Can you work these out from the model? Positions are in its coordinate system, mm. Face numbers are marked on the shaded views. A direction names the side the tool comes from. Round coordinates to 2 decimals unless told otherwise and drop trailing zeros. Loops run counter-clockwise (first coordinate to the right, second up) from the corner with the lowest first, then second, coordinate; pieces in that order, holes last.
(1) I want a section at C-C on x = 12. Write out the boundary of the cut face in (y, z), plus the area to 3 significant figures.
(2) I want a section at B-B on z = 3.75. Write out the boundary of the cut face in (x, y), plus the area to 3 significant figures.
(3) I want a section at A-A on x = 0. Write out the boundary of the cut face in (y, z), plus the area to 3 significant figures.
(4) Will these pins go through, and if not, where does the flat tip stop? pin 1 Ø4 at (x, y) = (0, 21) entering from +Z; pin 2 Ø4 at (x, z) = (9, 5.5) entering from -Y; pin 3 Ø2 at (x, z) = (-7.5, 12) entering from -Y.
(5) Which directions (+Z, -Z, +X, -X, +Y, -Y) give clear straight access to the entire face, cutting with the end or side of a thin tool? Please do the marked faces 1, 2, 3 and 4.
(6) I want a section at D-D on y = -6. Write out the boundary of the cut face in (x, z), plus the area to 3 significant figures.
(7) If I drill on line 1 along Y through (x, z) = (-12, 5.5); line 2 along Z through (x, y) = (-0.5, -0.5); line 3 along Y through (x, z) = (-3.5, 21.5), over which ranges is the centre line in solid material (lowest first)?
from build123d import *

# Parameters (mm, degrees)
F0_W         = 30
F0_H         = 60
F2_DEPTH     = 23
F3_DEPTH     = 10
F4_T1_DEPTH  = 135
F4_T3_DEPTH  = 105
F4_T8_DEPTH  = 105
F4_T14_DEPTH = 105
F4_T20_DEPTH = 105
F4_T27_DEPTH = 105
F4_T33_DEPTH = 105
F5_R         = 4


# Not quite as in the source:
# - a fillet or chamfer that OpenCascade refuses, or shapes differently, is made with other operations: its cross-section is extruded or revolved along the edge and cut away or added


with BuildPart() as f2:
    # F0 (on Top) → F2 (new body)
    with BuildSketch(Plane.XY):
        Rectangle(F0_W, F0_H)
    extrude(amount=F2_DEPTH)

    # F1 (on face) → F3 (join)
    with BuildSketch(Plane.XY):
        Polygon((4.8278798349, -30), (-4.8278798349, -30), (-4.8278798349, -56.4796291292), (0, -56.4796291292), (4.8278798349, -56.4796291292), align=None)
    extrude(amount=F3_DEPTH)

    # F4: fillet of radius 15 on 4 edges, made by hand

    # F4_s2 → F4_t1 (cut)
    with BuildSketch(Plane.XZ.offset(-67.5)):
        with BuildLine():
            ThreePointArc((-15, 8), (-10.6066017178, 18.6066017178), (0, 23))
            Line((0, 23), (-15, 23))
            Line((-15, 23), (-15, 8))
        make_face()
        with BuildLine():
            ThreePointArc((15, 8), (10.6066017178, 18.6066017178), (0, 23))
            Line((0, 23), (15, 23))
            Line((15, 23), (15, 8))
        make_face()
    extrude(amount=F4_T1_DEPTH, mode=Mode.SUBTRACT)

    # F4_s4 → F4_t3 (cut)
    with BuildSketch(Plane.YZ.offset(-52.5)):
        with BuildLine():
            ThreePointArc((30, 8), (25.6066017178, 18.6066017178), (15, 23))
            Line((15, 23), (30, 23))
            Line((30, 23), (30, 8))
        make_face()
    extrude(amount=F4_T3_DEPTH, mode=Mode.SUBTRACT)


with BuildPart() as f4_tool6:
    # F4_s7 → F4_t8 (new body)
    with BuildSketch(Plane.YZ.offset(-52.5)):
        with BuildLine():
            ThreePointArc((-15, 23), (-25.6066017178, 18.6066017178), (-30, 8))
            Line((-30, 8), (-30, 23))
            Line((-30, 23), (-15, 23))
        make_face()
    extrude(amount=F4_T8_DEPTH)

    split(bisect_by=Plane.YZ.offset(-4.8278798349), keep=Keep.BOTTOM)

    split(bisect_by=Plane.XY.offset(10), keep=Keep.TOP)


with BuildPart() as f2_1:
    add(f2.part)

    # F4_t5: cut F4_tool6
    add(f4_tool6.part, mode=Mode.SUBTRACT)


with BuildPart() as f4_tool12:
    # F4_s13 → F4_t14 (new body)
    with BuildSketch(Plane.YZ.offset(-52.5)):
        with BuildLine():
            ThreePointArc((-15, 23), (-25.6066017178, 18.6066017178), (-30, 8))
            Line((-30, 8), (-30, 23))
            Line((-30, 23), (-15, 23))
        make_face()
    extrude(amount=F4_T14_DEPTH)

    split(bisect_by=Plane.YZ.offset(-4.8278798349), keep=Keep.BOTTOM)

    split(bisect_by=Plane.XY.offset(10), keep=Keep.BOTTOM)


with BuildPart() as f2_2:
    add(f2_1.part)

    # F4_t11: cut F4_tool12
    add(f4_tool12.part, mode=Mode.SUBTRACT)


with BuildPart() as f4_tool18:
    # F4_s19 → F4_t20 (new body)
    with BuildSketch(Plane.YZ.offset(-52.5)):
        with BuildLine():
            ThreePointArc((-15, 23), (-25.6066017178, 18.6066017178), (-30, 8))
            Line((-30, 8), (-30, 23))
            Line((-30, 23), (-15, 23))
        make_face()
    extrude(amount=F4_T20_DEPTH)

    split(bisect_by=Plane.YZ.offset(-4.8278798349), keep=Keep.TOP)

    split(bisect_by=Plane.XY.offset(10), keep=Keep.TOP)

    split(bisect_by=Plane.YZ.offset(4.8278798349), keep=Keep.BOTTOM)


with BuildPart() as f2_3:
    add(f2_2.part)

    # F4_t17: cut F4_tool18
    add(f4_tool18.part, mode=Mode.SUBTRACT)


with BuildPart() as f4_tool25:
    # F4_s26 → F4_t27 (new body)
    with BuildSketch(Plane.YZ.offset(-52.5)):
        with BuildLine():
            ThreePointArc((-15, 23), (-25.6066017178, 18.6066017178), (-30, 8))
            Line((-30, 8), (-30, 23))
            Line((-30, 23), (-15, 23))
        make_face()
    extrude(amount=F4_T27_DEPTH)

    split(bisect_by=Plane.XY.offset(10), keep=Keep.TOP)

    split(bisect_by=Plane.YZ.offset(4.8278798349), keep=Keep.TOP)


with BuildPart() as f2_4:
    add(f2_3.part)

    # F4_t24: cut F4_tool25
    add(f4_tool25.part, mode=Mode.SUBTRACT)


with BuildPart() as f4_tool31:
    # F4_s32 → F4_t33 (new body)
    with BuildSketch(Plane.YZ.offset(-52.5)):
        with BuildLine():
            ThreePointArc((-15, 23), (-25.6066017178, 18.6066017178), (-30, 8))
            Line((-30, 8), (-30, 23))
            Line((-30, 23), (-15, 23))
        make_face()
    extrude(amount=F4_T33_DEPTH)

    split(bisect_by=Plane.XY.offset(10), keep=Keep.BOTTOM)

    split(bisect_by=Plane.YZ.offset(4.8278798349), keep=Keep.TOP)


with BuildPart() as f2_5:
    add(f2_4.part)

    # F4_t30: cut F4_tool31
    add(f4_tool31.part, mode=Mode.SUBTRACT)

    # F5
    f5_edges = [f2_5.edges().sort_by_distance(p)[0] for p in [
        (-4.82788, -43.172849, 10),
        (4.82788, -43.172849, 10),
        (0, -56.479629, 10),
    ]]
    fillet(f5_edges, radius=F5_R)


solid = f2_5.part
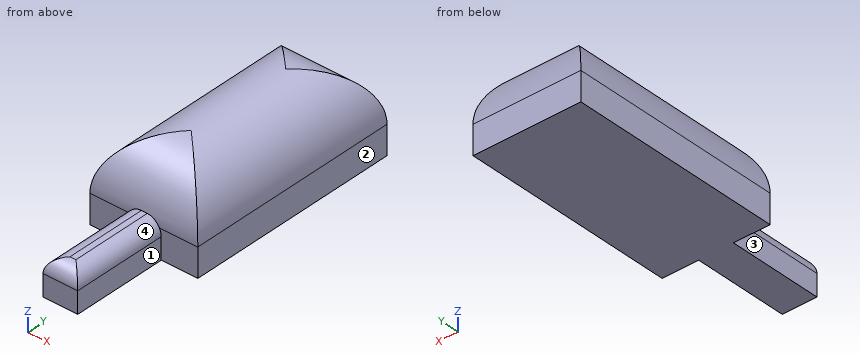
Filled sheet:
1. outline: (-30, 0) - (30, 0) - (30, 8) arc R15 ccw to (27, 17) - (-27, 17) arc R15 ccw to (-30, 8) - close
1. area: 1,000 mm2
2. outline: (-15, -30) - (-4.83, -30) - (-4.83, -56.48) - (4.83, -56.48) - (4.83, -30) - (15, -30) - (15, 30) - (-15, 30) - close
2. area: 2,060 mm2
3. outline: (-56.48, 0) - (30, 0) - (30, 8) arc R15 ccw to (15, 23) - (-15, 23) arc R15 ccw to (-29.87, 10) - (-52.48, 10) arc R4 ccw to (-56.48, 6) - close
3. area: 1,540 mm2
4. pin 1: stops at z = 22.46
4. pin 2: stops at y = -30
4. pin 3: stops at y = -29.7
5. face 1: +Z, -Z, +X, -Y
5. face 2: +Z, -Z, +X, +Y, -Y
5. face 3: +Z, -Z, -X, -Y
5. face 4: +Z, +X, -Y
6. outline: (-15, 0) - (15, 0) - (15, 8) arc R15 ccw to (-15, 8) - close
6. area: 593 mm2
7. line 1: y = -30 to 30
7. line 2: z = 0 to 22.99
7. line 3: y = -21.54 to 21.54
